Design review of the part built by this model. Coordinates are the model's own, in mm. A direction names the side the tool comes from. Coordinates: 2 decimals unless noted, no trailing zeros. Order: outer loops, then holes, each group sorted by start corner. A loop starts at its lowest first (then second) coordinate and runs counter-clockwise, first axis right, second up. Notation, with made-up numbers: M 85.5,2.5 L 135.5,2.5 A19 ccw 135.5,32.5 Z; hole C 1.5,32.5 d1. An arc over 180 degrees is marked long. Answer in a Markdown table with one row per item.
from build123d import *
from build123d.topology import SkipClean

# Parameters (mm, degrees)
SKETCH3_R               = 3
CUT_EXTRUDE1_DEPTH      = 48.754580932
SKETCH4_W               = 8
SKETCH4_H               = 1
BOSS_EXTRUDE1_DEPTH     = 6
BOSS_EXTRUDE2_START     = 6
SKETCH5_W               = 18
SKETCH5_H               = 18
BOSS_EXTRUDE2_DEPTH     = 6
BOSS_EXTRUDE3_START     = 1
SKETCH13_R              = 4
BOSS_EXTRUDE3_DEPTH     = 1
CHAMFER1_SIZE           = 6
CHAMFER2_SIZE2          = 1
CHAMFER2_SIZE           = 2.747477419
CUT_EXTRUDE2_DEPTH      = 49.872282533
CUT_EXTRUDE2_DEPTH_BACK = 49.872282533
SKETCH6_W               = 1
SKETCH6_H               = 36
CUT_EXTRUDE5_DEPTH      = 49.420037175
CUT_EXTRUDE5_DEPTH_BACK = 49.420037175
SKETCH7_R               = 1.55
CUT_EXTRUDE6_START      = 9
CUT_EXTRUDE6_DEPTH      = 40.420037195
CUT_EXTRUDE7_START      = 9
SKETCH9_R               = 3.1
CUT_EXTRUDE7_DEPTH      = 40.420037195
SKETCH11_R              = 2.5
BODY_MOVE_COPY1_ANGLE   = 180


with BuildPart() as part:
    # Sketch2 → Revolve1 (revolve)
    with BuildSketch(Plane(origin=(0, 0, 0), x_dir=(1, 0, 0), z_dir=(0, 1, 0))):
        with BuildLine():
            Line((0, 0), (0, 3))
            Line((0, 3), (33.5, 3))
            Line((33.5, 3), (33.5, 2.5))
            ThreePointArc((33.5, 2.5), (31, 0), (33.5, -2.5))
            Line((33.5, -2.5), (33.5, -3))
            Line((33.5, -3), (0, -3))
            Line((0, -3), (0, 0))
        make_face()
    revolve(axis=Axis((0, 0, 0), (0, 0, -1)))

    # Sketch3 → Cut-Extrude1 (cut, through all)
    with BuildSketch(Plane(origin=(0, 0, -3), x_dir=(-1, 0, 0), z_dir=(0, 0, -1))):
        Circle(SKETCH3_R)
    extrude(amount=-CUT_EXTRUDE1_DEPTH, mode=Mode.SUBTRACT)

    # Sketch4 → Boss-Extrude1 (add)
    with BuildSketch(Plane(origin=(0, 0, -3), x_dir=(-1, 0, 0), z_dir=(0, 0, -1))):
        with Locations((0, 3)):
            Rectangle(SKETCH4_W, SKETCH4_H)
    extrude(amount=-BOSS_EXTRUDE1_DEPTH)

    # Sketch5 → Boss-Extrude2 (add)
    with BuildSketch(Plane(origin=(0, 0, -3), x_dir=(-1, 0, 0), z_dir=(0, 0, -1)).offset(BOSS_EXTRUDE2_START)):
        Rectangle(SKETCH5_W, SKETCH5_H)
        with BuildLine():
            Line((-1.658312395, 2.5), (1.658312395, 2.5))
            ThreePointArc((1.658312395, 2.5), (0, -3), (-1.658312395, 2.5))
        make_face(mode=Mode.SUBTRACT)
    extrude(amount=-BOSS_EXTRUDE2_DEPTH)

    # Sketch13 → Boss-Extrude3 (add)
    with SkipClean():  # the faces are left unmerged after this step: merging them gives an invalid solid
        with BuildSketch(Plane(origin=(0, 0, -9), x_dir=(-1, 0, 0), z_dir=(0, 0, -1)).offset(BOSS_EXTRUDE3_START)):
            Circle(SKETCH13_R)
            with BuildLine():
                Line((1.658312395, 2.5), (-1.658312395, 2.5))
                ThreePointArc((-1.658312395, 2.5), (-1.833910419, 2.374188825), (-2, 2.236067977))
                Line((-2, 2.236067977), (-2, -2.236067977))
                ThreePointArc((-2, -2.236067977), (0, -3), (2, -2.236067977))
                Line((2, -2.236067977), (2, 2.236067977))
                ThreePointArc((2, 2.236067977), (1.833910419, 2.374188825), (1.658312395, 2.5))
            make_face(mode=Mode.SUBTRACT)
        extrude(amount=-BOSS_EXTRUDE3_DEPTH)

    # Chamfer1
    chamfer1_edges = [part.edges().sort_by_distance(p)[0] for p in [
        (0, -9, -3),
        (0, 9, -3),
        (9, 0, -3),
        (-9, 0, -3),
    ]]
    chamfer(chamfer1_edges, length=CHAMFER1_SIZE - 0.0001)  # a hair under: the kernel refuses the full size

    # Chamfer2
    chamfer2_edges = [part.edges().sort_by_distance(p)[0] for p in [
        (4, 0, -9),
    ]]
    chamfer2_side = [part.faces().sort_by_distance(p)[0] for p in [
        (4.02, 0, -9),
    ]]
    chamfer(chamfer2_edges, length=CHAMFER2_SIZE - 0.0001, length2=CHAMFER2_SIZE2 - 0.0001, reference=chamfer2_side[0])  # a hair under: the kernel refuses the full size

    # Sketch6 → Cut-Extrude2 (cut, two sides: drawn at the far end of the back side and taken through both)
    with BuildSketch(Plane(origin=(0, 0, -9), x_dir=(-1, 0, 0), z_dir=(0, 0, -1)).offset(-CUT_EXTRUDE2_DEPTH_BACK)):
        Rectangle(SKETCH6_W, SKETCH6_H)
    extrude(amount=CUT_EXTRUDE2_DEPTH + CUT_EXTRUDE2_DEPTH_BACK, mode=Mode.SUBTRACT)

    # Sketch7 → Cut-Extrude5 (cut, two sides: drawn at the far end of the back side and taken through both)
    with BuildSketch(Plane.ZY.offset(-CUT_EXTRUDE5_DEPTH_BACK)):
        with Locations((-6.2, 4)):
            Circle(SKETCH7_R)
        with Locations(Location((-6.2, -4.5, 0), (0, 0, 84.161721877))):
            Circle(SKETCH7_R)
    extrude(amount=CUT_EXTRUDE5_DEPTH + CUT_EXTRUDE5_DEPTH_BACK, mode=Mode.SUBTRACT)

    # Sketch8 → Cut-Extrude6 (cut, through all)
    with BuildSketch(Plane(origin=(0, 0, 0), x_dir=(0, 0, -1), z_dir=(1, 0, 0)).offset(CUT_EXTRUDE6_START)):
        Polygon((6.2, 7.233161507), (3.4, 5.616580754), (3.4, 2.383419246), (6.2, 0.766838493), (9, 2.383419246), (9, 5.616580754), align=None)
        Polygon((9, -2.883419246), (6.2, -1.266838493), (3.4, -2.883419246), (3.4, -6.116580754), (6.2, -7.733161507), (9, -6.116580754), align=None)
    extrude(amount=CUT_EXTRUDE6_DEPTH, mode=Mode.SUBTRACT)

    # Sketch9 → Cut-Extrude7 (cut, through all)
    with BuildSketch(Plane.ZY.offset(CUT_EXTRUDE7_START)):
        with Locations((-6.2, 4)):
            Circle(SKETCH9_R)
        with Locations((-6.2, -4.5)):
            Circle(SKETCH9_R)
    extrude(amount=CUT_EXTRUDE7_DEPTH, mode=Mode.SUBTRACT)


with BuildPart() as body_2:
    # Sketch11 → Revolve2 (revolve)
    with BuildSketch(Plane(origin=(0, 0, 0), x_dir=(1, 0, 0), z_dir=(0, 1, 0)), mode=Mode.PRIVATE) as revolve2_sk:
        with Locations((33.5, 0)):
            Circle(SKETCH11_R)
    revolve(revolve2_sk.sketch.rotate(Axis((0, 0, 0), (0, 0, 1)), 180), axis=Axis((0, 0, 0), (0, 0, 1)))


with BuildPart() as part_1:
    # Body-Move/Copy1: read off the stored shape, not the designer's step
    # Body-Move/Copy1: moved
    add(part.part.moved(Location((0.5, -8.5, -3))).rotate(Axis((0, 0, 0), (0.7071067812, -0.7071067812, 0)), BODY_MOVE_COPY1_ANGLE))


solid = part_1.part
(1) Insertion check: pin 1 Ø1 at (x, y) = (-5, -21.5) entering from +Z; pin 2 Ø5 at (y, z) = (-21, 3.5) entering from +X; pin 3 Ø6.5 at (x, z) = (0, 8.5) entering from +Y; pin 4 Ø1.9 at (x, z) = (13, 9.2) entering from +Y. Each pin has a flat end and moves straight along its axis. Give the tip position at first contact, or say it passes through.
Return value:
| item | result |
|---|---|
| pin 1 | stops at z = 6 |
| pin 2 | stops at x = 36.09 |
| pin 3 | stops at y = 32.38 |
| pin 4 | passes through |
(2) Draft analysis for pull direction X (two halves, no side actions). For faces 1 (the flat face through (20.5, 5.5, 9)), 2 (the cylindrical face through (-24.203, 6.762, 5.747)), 3 (the cylindrical face through (2.963, -5.309, 9.402)), state which applies: pulls with the +X half, pulls with the -X half, needs draft (parallel to the pull), parting line crosses it, or undercut.
Return value:
| item | result |
|---|---|
| face 1 | pulls with the +X half |
| face 2 | parting line crosses it |
| face 3 | undercut |
(3) Add section A-A, the plane z = 2.5. Give the boundary of the cut face in (x, y).
Return value:
| item | result |
|---|---|
| outline | C 8.5,-0.5 d62.1; hole M -9.5,-1 L 6,-1 L 6,-2.16 A3 ccw 11.46,-1 L 26.5,-1 L 26.5,0 L 11.46,0 A3 ccw 6,1.16 L 6,0 L -9.5,0 Z |
(4) For line 1 along X through (y, z) = (10.2, 9.2); line 2 along Z through (x, y) = (26, -29); line 3 along Z through (x, y) = (13, 5), list the stretches that pass through material, from the lowest coordinate up. Write a range as from..to.
Return value:
| item | result |
|---|---|
| line 1 | x = -3.3..1.4, 7.6..9.9, 16.1..20.3 |
| line 2 | z = 0..0.5, 5.5..6 |
| line 3 | z = 0..7.65, 10.75..12 |
(5) For faces 4 (the flat face through (0, -1, 5)), 5 (the flat face through (2.064, -11.639, 7.82)), 6 (the flat face through (4, -12, 6.4)), list the 3-axis set-ups (+Z, -Z, +X, -X, +Y, -Y) from which the entire face can be reached by the end or side of a thin tool; tool diameter is ignored.
Return value:
| item | result |
|---|---|
| face 4 | +Z, -Z |
| face 5 | -Y |
| face 6 | +Z, -Y |
